Source: CAD feature listing. Evaluate the final solid. Frame: model axes, mm. Face numbers are marked on the shaded views. A direction names the side the tool comes from. Coordinates: 2 decimals unless noted, no trailing zeros. Write each loop counter-clockwise with the first axis right and the second up, starting at its lowest first coordinate (ties: lowest second). Pieces come first, ordered by that corner, then holes. Notation, with made-up numbers: M 42.25,-10.75 L 52.25,-10.75 A31 cw 52.25,25.25 Z; hole C -26,-19.75 d6. An arc over 180 degrees is marked long. One line per item, written item: value. Start each with the question number.
Item 1: Set-up query: the marked faces 4 and 5. Return all of +Z, -Z, +X, -X, +Y, -Y with unobstructed straight access to the full face (end or side cutting, diameter ignored); none if empty.
Item 2: Cut plane A-A, the plane y = 8.25. Output: boundary loops of the cut face in (x, z).
Item 3: Cut plane B-B, the plane x = -20. Output: boundary loops of the cut face in (y, z), then the cut area to 3 significant figures.
Item 4: Cut plane C-C, the plane z = 20. Output: boundary loops of the cut face in (x, y), then the cut area to 3 significant figures.
Item 5: Mould query, pull axis X, two halves, no side actions, for the marked faces 1, 2 and 3. Classes: released by +X, released by -X, zero draft, split by the parting line, or undercut.
Item 6: Ray query, L1, parallel to Z at x = 0, y = 9; L2, parallel to Z at x = -20, y = 14.75; L3, parallel to Z at x = -20, y = 6.5. Return the intervals inside material, ascending. Write a range as from..to.
Item 7: Pin query (flat end, axial travel): P1, Ø7.5, axis at x = -22, z = 23, coming from the +Y side; P2, Ø6.5, axis at x = 0, z = 0, coming from the +Y side. Return the tip coordinate at first contact, or that it passes through.
Item 8: Cut plane D-D, the plane x = 0.5. Output: boundary loops of the cut face in (y, z), then the cut area to 3 significant figures.
```python
from build123d import *

# Parameters (mm, degrees)
SZKIC1_W                                            = 80
SZKIC1_H                                            = 80
DODANIE_WYCI_GNI_CIE1_DEPTH                         = 20
POG_BIENIE_WALCOWE_POD_M8_WKR_T_Z_BEM_W_D           = 9
POG_BIENIE_WALCOWE_POD_M8_WKR_T_Z_BEM_W_CBORE_D     = 15
POG_BIENIE_WALCOWE_POD_M8_WKR_T_Z_BEM_W_CBORE_DEPTH = 8.6
OTWORY_USTALAJ_CE_8_0MM1_D                          = 8
ZAOKR_GLENIE1_R                                     = 10


with BuildPart() as part:
    # Szkic1 → Dodanie-wyciągnięcie1 (new body)
    with BuildSketch(Plane(origin=(0, 0, 0), x_dir=(1, 0, 0), z_dir=(0, 1, 0))):
        Rectangle(SZKIC1_W, SZKIC1_H)
    extrude(amount=DODANIE_WYCI_GNI_CIE1_DEPTH)

    # Pogłębienie walcowe pod M8 Wkręt z łbem walcowym z gniazdem sześciokątnym1 (through all)
    with Locations(Plane(origin=(0, 20, 0), x_dir=(1, 0, 0), z_dir=(0, 1, 0))):
        with Locations((-20, 20), (20, 20), (20, -20), (-20, -20)):
            CounterBoreHole(POG_BIENIE_WALCOWE_POD_M8_WKR_T_Z_BEM_W_D / 2, POG_BIENIE_WALCOWE_POD_M8_WKR_T_Z_BEM_W_CBORE_D / 2, POG_BIENIE_WALCOWE_POD_M8_WKR_T_Z_BEM_W_CBORE_DEPTH)

    # Otwory ustalające Ø8.0mm1 (through all)
    with Locations(Plane(origin=(0, 20, 0), x_dir=(1, 0, 0), z_dir=(0, 1, 0))):
        with Locations((0, 27), (0, 0), (0, -27)):
            Hole(OTWORY_USTALAJ_CE_8_0MM1_D / 2)

    # Zaokrąglenie1
    zaokr_glenie1_edges = [part.edges().sort_by_distance(p)[0] for p in [
        (40, 10, 40),
        (-40, 10, 40),
        (-40, 10, -40),
        (40, 10, -40),
    ]]
    fillet(zaokr_glenie1_edges, radius=ZAOKR_GLENIE1_R)


solid = part.part
```
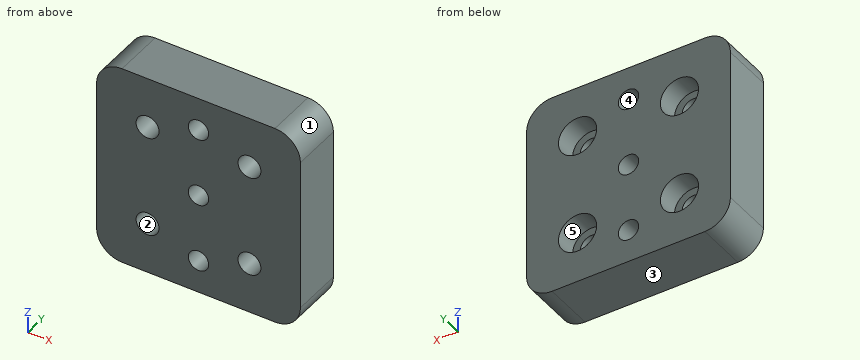
From the geometry:
1. face 4: +Y, -Y
1. face 5: +Y
2. outline: M -40,-30 A10 ccw -30,-40 L 30,-40 A10 ccw 40,-30 L 40,30 A10 ccw 30,40 L -30,40 A10 ccw -40,30 Z; hole C -20,-20 d9; hole C -20,20 d9; hole C 0,-27 d8; hole C 0,0 d8; hole C 0,27 d8; hole C 20,-20 d9; hole C 20,20 d9
3. outline: M 0,-40 L 20,-40 L 20,-27.5 L 11.4,-27.5 L 11.4,-24.5 L 0,-24.5 Z; M 0,-15.5 L 11.4,-15.5 L 11.4,-12.5 L 20,-12.5 L 20,12.5 L 11.4,12.5 L 11.4,15.5 L 0,15.5 Z; M 0,24.5 L 11.4,24.5 L 11.4,27.5 L 20,27.5 L 20,40 L 0,40 Z
3. area: 1,140 mm²
4. outline: M -40,0 L -24.5,0 L -24.5,11.4 L -27.5,11.4 L -27.5,20 L -40,20 Z; M -15.5,0 L 15.5,0 L 15.5,11.4 L 12.5,11.4 L 12.5,20 L -12.5,20 L -12.5,11.4 L -15.5,11.4 Z; M 24.5,0 L 40,0 L 40,20 L 27.5,20 L 27.5,11.4 L 24.5,11.4 Z
4. area: 1,140 mm²
5. face 1: released by +X
5. face 2: undercut
5. face 3: zero draft
6. L1: z = -40..-31, -23..-4, 4..23, 31..40
6. L2: z = -40..-27.5, -12.5..12.5, 27.5..40
6. L3: z = -40..-24.5, -15.5..15.5, 24.5..40
7. P1: stops at y = 11.4
7. P2: passes through
8. outline: M 0,-40 L 20,-40 L 20,-30.97 L 0,-30.97 Z; M 0,-23.03 L 20,-23.03 L 20,-3.97 L 0,-3.97 Z; M 0,3.97 L 20,3.97 L 20,23.03 L 0,23.03 Z; M 0,30.97 L 20,30.97 L 20,40 L 0,40 Z
8. area: 1,120 mm²
